from build123d import *

# Parameters (mm, degrees)
SKETCH1_R                                      = 10.5664
BOSS_EXTRUDE1_DEPTH                            = 4.7752
CIRPATTERN1_COUNT                              = 4
CSK_FOR_6_FLAT_HEAD_MACHINE_SCREW1_D           = 3.6576
CSK_FOR_6_FLAT_HEAD_MACHINE_SCREW1_CSINK_D     = 7.0866
CSK_FOR_6_FLAT_HEAD_MACHINE_SCREW1_CSINK_ANGLE = 82
CUT_EXTRUDE1_DEPTH                             = 1.3716


with BuildPart() as part:
    # Sketch1 → Boss-Extrude1 (new body)
    with BuildSketch(Plane.XY):
        with BuildLine():
            Line((-20.6502, 25.273), (20.6502, 25.273))
            ThreePointArc((20.6502, 25.273), (28.685169884, 22.769919997), (33.876987837, 16.146387942))
            Line((33.876987837, 16.146387942), (39.16808693, 2.208601518))
            ThreePointArc((39.16808693, 2.208601518), (39.5732, 0), (39.16808693, -2.208601518))
            Line((39.16808693, -2.208601518), (33.876987837, -16.146387942))
            ThreePointArc((33.876987837, -16.146387942), (28.685169884, -22.769919997), (20.6502, -25.273))
            Line((20.6502, -25.273), (-20.6502, -25.273))
            ThreePointArc((-20.6502, -25.273), (-28.685169884, -22.769919997), (-33.876987837, -16.146387942))
            Line((-33.876987837, -16.146387942), (-39.16808693, -2.208601518))
            ThreePointArc((-39.16808693, -2.208601518), (-39.5732, 0), (-39.16808693, 2.208601518))
            Line((-39.16808693, 2.208601518), (-33.876987837, 16.146387942))
            ThreePointArc((-33.876987837, 16.146387942), (-28.685169884, 22.769919997), (-20.6502, 25.273))
        make_face()
        Circle(SKETCH1_R, mode=Mode.SUBTRACT)
    extrude(amount=-BOSS_EXTRUDE1_DEPTH)

    # Sketch2 → #4-40 Tapped Hole1 (revolve, cut)
    with BuildSketch(Plane(origin=(11.5062, 11.5062, 0), x_dir=(0, -1, 0), z_dir=(1, 0, 0))):
        Polygon((0, 0), (0, 4.7752), (1.6764, 4.7752), (1.1303, 4.2291), (1.1303, 0.5461), (1.6764, 0), align=None)
    f_4_40_tapped_hole1 = revolve(axis=Axis((11.5062, 11.5062, 6.35), (0, 0, -1)), mode=Mode.SUBTRACT)

    # CirPattern1: #4-40 Tapped Hole1 ×4 about axis
    cirpattern1_axis = Axis((0, 0, 0), (0, 0, 1))
    for i in range(1, CIRPATTERN1_COUNT):
        add(f_4_40_tapped_hole1.rotate(cirpattern1_axis, i * 360 / CIRPATTERN1_COUNT), mode=Mode.SUBTRACT)

    # CSK for #6 Flat Head Machine Screw1 (through all)
    with Locations(Plane.XY):
        with Locations((33.3502, 0), (-33.3502, 0)):
            CounterSinkHole(CSK_FOR_6_FLAT_HEAD_MACHINE_SCREW1_D / 2, CSK_FOR_6_FLAT_HEAD_MACHINE_SCREW1_CSINK_D / 2, counter_sink_angle=CSK_FOR_6_FLAT_HEAD_MACHINE_SCREW1_CSINK_ANGLE)

    # Sketch6 → Cut-Extrude1 (cut)
    with BuildSketch(Plane.XY):
        with BuildLine():
            Line((23.7617, 11.5062), (23.7617, -11.5062))
            ThreePointArc((23.7617, -11.5062), (20.172147157, -20.172147157), (11.5062, -23.7617))
            Line((11.5062, -23.7617), (-11.5062, -23.7617))
            ThreePointArc((-11.5062, -23.7617), (-20.172147157, -20.172147157), (-23.7617, -11.5062))
            Line((-23.7617, -11.5062), (-23.7617, 11.5062))
            ThreePointArc((-23.7617, 11.5062), (-20.172147157, 20.172147157), (-11.5062, 23.7617))
            Line((-11.5062, 23.7617), (11.5062, 23.7617))
            ThreePointArc((11.5062, 23.7617), (20.172147157, 20.172147157), (23.7617, 11.5062))
        make_face()
        with BuildLine():
            Line((21.0439, 11.5062), (21.0439, -11.5062))
            ThreePointArc((21.0439, -11.5062), (18.250372347, -18.250372347), (11.5062, -21.0439))
            Line((11.5062, -21.0439), (-11.5062, -21.0439))
            ThreePointArc((-11.5062, -21.0439), (-18.250372347, -18.250372347), (-21.0439, -11.5062))
            Line((-21.0439, -11.5062), (-21.0439, 11.5062))
            ThreePointArc((-21.0439, 11.5062), (-18.250372347, 18.250372347), (-11.5062, 21.0439))
            Line((-11.5062, 21.0439), (11.5062, 21.0439))
            ThreePointArc((11.5062, 21.0439), (18.250372347, 18.250372347), (21.0439, 11.5062))
        make_face(mode=Mode.SUBTRACT)
    extrude(amount=-CUT_EXTRUDE1_DEPTH, mode=Mode.SUBTRACT)


solid = part.part
Source: CAD feature listing. Evaluate the final solid. Frame: model axes, mm. A direction names the side the tool comes from. Round coordinates to 2 decimals unless told otherwise and drop trailing zeros. Loops run counter-clockwise (first coordinate to the right, second up) from the corner with the lowest first, then second, coordinate; pieces in that order, holes last.
Q1. Section D-D, the plane y = 6. Return loops of the section in (x, z).
Q2. Section A-A, the plane y = 0. Return loops of the section in (x, z), plus the area to 3 significant figures.
Q3. Access query for faces 4 (the face through (5, 10, 0)), 5 (the face through (20.076, 20.267, -0.676)). Directions: +Z, -Z, +X, -X, +Y, -Y. A direction counts if a zero-diameter tool reaches every point of the face in a straight line with its end or side. Return the directions, or none.
Q4. Section C-C, the plane x = 0. Return loops of the section in (y, z).
Q5. Mould query, pull axis X, two halves, no side actions, for faces 1 (the face through (-31.523, 0.08, -3.393)), 2 (the face through (9.35, -5.26, -4.775)), 3 (the face through (-36.485, -9.275, -2.354)). Classes: pulls with the +X half, pulls with the -X half, needs draft (parallel to the pull), parting line crosses it, or undercut.
Q6. Section B-B, the plane z = -3.2. Return loops of the section in (x, y).
Q7. Ray query, line 1 (X direction, y = 8.5, z = -1.1); line 2 (X direction, y = -1, z = -0.55); line 3 (X direction, y = 6.5, z = -0.75). Return the intervals inside material, ascending.
Q8. First-contact query: P1, Ø0.7, axis at y = -3, z = -1, coming from the +X side; P2, Ø1.1, axis at y = 1, z = -1, coming from the +X side; P3, Ø2.5, axis at x = 11.51, y = 11.51, coming from the +Z side. Flat tips, straight axial feed; report the tip coordinate or a pass-through.
Solutions:
1. outline: (-37.73, -4.78) - (-8.7, -4.78) - (-8.7, 0) - (-21.04, 0) - (-21.04, -1.37) - (-23.76, -1.37) - (-23.76, 0) - (-37.73, 0) - close; (8.7, -4.78) - (37.73, -4.78) - (37.73, 0) - (23.76, 0) - (23.76, -1.37) - (21.04, -1.37) - (21.04, 0) - (8.7, 0) - close
2. outline: (-39.57, -4.78) - (-35.18, -4.78) - (-35.18, -1.97) - (-36.89, 0) - (-39.57, 0) - close; (-31.52, -4.78) - (-10.57, -4.78) - (-10.57, 0) - (-21.04, 0) - (-21.04, -1.37) - (-23.76, -1.37) - (-23.76, 0) - (-29.81, 0) - (-31.52, -1.97) - close; (10.57, -4.78) - (31.52, -4.78) - (31.52, -1.97) - (29.81, 0) - (23.76, 0) - (23.76, -1.37) - (21.04, -1.37) - (21.04, 0) - (10.57, 0) - close; (35.18, -4.78) - (39.57, -4.78) - (39.57, 0) - (36.89, 0) - (35.18, -1.97) - close
2. area: 228 mm2
3. face 4: +Z, +X, -X, +Y, -Y
3. face 5: +Z
4. outline: (-25.27, -4.78) - (-10.57, -4.78) - (-10.57, 0) - (-21.04, 0) - (-21.04, -1.37) - (-23.76, -1.37) - (-23.76, 0) - (-25.27, 0) - close; (10.57, -4.78) - (25.27, -4.78) - (25.27, 0) - (23.76, 0) - (23.76, -1.37) - (21.04, -1.37) - (21.04, 0) - (10.57, 0) - close
5. face 1: undercut
5. face 2: needs draft
5. face 3: pulls with the -X half
6. outline: (-39.17, -2.21) - (-33.88, -16.15) arc R14.15 ccw to (-20.65, -25.27) - (20.65, -25.27) arc R14.15 ccw to (33.88, -16.15) - (39.17, -2.21) arc R6.22 ccw to (39.17, 2.21) - (33.88, 16.15) arc R14.15 ccw to (20.65, 25.27) - (-20.65, 25.27) arc R14.15 ccw to (-33.88, 16.15) - (-39.17, 2.21) arc R6.22 ccw to start; hole circle Ø3.66 at (-33.35, 0); hole circle Ø2.26 at (-11.51, -11.51); hole circle Ø2.26 at (-11.51, 11.51); hole circle Ø21.13 at (0, 0); hole circle Ø2.26 at (11.51, -11.51); hole circle Ø2.26 at (11.51, 11.51); hole circle Ø3.66 at (33.35, 0)
7. line 1: x = -36.78 to -23.76, -21.04 to -6.28, 6.28 to 21.04, 23.76 to 36.78
7. line 2: x = -39.49 to -36.25, -30.45 to -23.76, -21.04 to -10.52, 10.52 to 21.04, 23.76 to 30.45, 36.25 to 39.49
7. line 3: x = -37.54 to -23.76, -21.04 to -8.33, 8.33 to 21.04, 23.76 to 37.54
8. P1: stops at x = 39
8. P2: stops at x = 39.56
8. P3: stops at z = -0.42
